Input: part model. Units: mm. Frame: model coordinates. A direction names the side the tool comes from. Round coordinates to 2 decimals unless told otherwise and drop trailing zeros. Loops run counter-clockwise (first coordinate to the right, second up) from the corner with the lowest first, then second, coordinate; pieces in that order, holes last.
(1) Line query: line 1 (X direction, y = -3.5, z = 1.1); line 2 (X direction, y = -6, z = 0.45); line 3 (Y direction, x = 0, z = 1.5). Output: solid intervals per line, ascending.
(2) Cut plane D-D, the plane x = 40. Output: boundary loops of the cut face in (y, z), and give its area (3 significant figures).
(3) Access query for faces 3 (the face through (8, -8, 1)), 4 (the face through (25, -3, 1.5)), 5 (the face through (23, -6, 1)), 6 (the face through (32, 0.1, 0.8)). Directions: +Z, -Z, +X, -X, +Y, -Y. A direction counts if a zero-diameter tool reaches every point of the face in a straight line with its end or side. Return the directions, or none.
(4) Cut plane A-A, the plane y = -6. Output: boundary loops of the cut face in (x, z), and give its area (3 significant figures).
(5) Draft query along X for faces 1 (the face through (9.5, 3, 1.5)), 2 (the face through (-1.97, -4.63, 0.99)). Return one class per face: released by +X, released by -X, zero draft, split by the parting line, or undercut.
(6) Cut plane B-B, the plane z = 1.35. Give the number of separate pieces and of enclosed holes in the cut face, and give its area (3 significant figures).
(7) First-contact query: pin 1 Ø1.6 at (x, y) = (0, 6) entering from -Z; pin 2 Ø1.1 at (x, z) = (21.5, 0.5) entering from -Y; pin 3 Ø0.6 at (y, z) = (-5, 1.5) entering from +X; pin 4 Ø3 at (x, y) = (19.5, -0.5) entering from +Z. Flat tips, straight axial feed; report the tip coordinate or a pass-through.
(8) Cut plane C-C, the plane x = 35. Output: boundary loops of the cut face in (y, z), and give its area (3 significant figures).
from build123d import *

# Parameters (mm, degrees)
CROQUIS1_R              = 0.9
CROQUIS1_R_2            = 1.1
SALIENTE_EXTRUIR1_DEPTH = 2
CROQUIS2_W              = 12
CROQUIS2_H              = 3
CORTAR_EXTRUIR1_DEPTH   = 1
CROQUIS3_W              = 6
CROQUIS3_H              = 10
CORTAR_EXTRUIR2_DEPTH   = 44.194444087


with BuildPart() as part:
    # Croquis1 → Saliente-Extruir1 (new body)
    with BuildSketch(Plane.XY):
        with BuildLine():
            Line((-1.326649916, 8), (20, 8))
            Line((20, 8), (20, 0))
            Line((20, 0), (8, 0))
            Line((8, 0), (8, 4))
            Line((8, 4), (1.326649916, 4))
            ThreePointArc((1.326649916, 4), (-2, 4.673350084), (-1.326649916, 8))
        make_face()
        with Locations((0, 6)):
            Circle(CROQUIS1_R, mode=Mode.SUBTRACT)
        with Locations((12, 3.5)):
            Circle(CROQUIS1_R_2, mode=Mode.SUBTRACT)
    extrude(amount=SALIENTE_EXTRUIR1_DEPTH)

    # Croquis2 → Cortar-Extruir1 (cut)
    with BuildSketch(Plane.XY.offset(2)):
        with Locations((14, 1.5)):
            Rectangle(CROQUIS2_W, CROQUIS2_H)
    extrude(amount=-CORTAR_EXTRUIR1_DEPTH, mode=Mode.SUBTRACT)

    # Simetría1: part across plane


with BuildPart() as part_1:
    add(part.part)
    add(part.part.mirror(Plane(origin=(20, 0, 2), x_dir=(0, 0, 1), z_dir=(0, 1, 0))))

    # Simetría2: part across plane


with BuildPart() as part_2:
    add(part_1.part)
    add(part_1.part.mirror(Plane(origin=(20, 8, 2), x_dir=(0, 0, 1), z_dir=(-1, 0, 0))))

    # Croquis3 → Cortar-Extruir2 (cut, through all)
    with BuildSketch(Plane.XY.offset(2)):
        with Locations((20, -8)):
            Rectangle(CROQUIS3_W, CROQUIS3_H)
    extrude(amount=-CORTAR_EXTRUIR2_DEPTH, mode=Mode.SUBTRACT)


solid = part_2.part
Reported:
1. line 1: x = 8 to 10.9, 13.1 to 17, 23 to 26.9, 29.1 to 32
1. line 2: x = -2.4 to -0.9, 0.9 to 17, 23 to 39.1, 40.9 to 42.4
1. line 3: y = -8 to -6.9, -5.1 to -3.6, 3.6 to 5.1, 6.9 to 8
2. outline: (-8, 0) - (-6.9, 0) - (-6.9, 2) - (-8, 2) - close; (-5.1, 0) - (-3.6, 0) - (-3.6, 2) - (-5.1, 2) - close; (3.6, 0) - (5.1, 0) - (5.1, 2) - (3.6, 2) - close; (6.9, 0) - (8, 0) - (8, 2) - (6.9, 2) - close
2. area: 10.4 mm2
3. face 3: +Z, -Z, +X, -X, -Y
3. face 4: +Z, +X, -X
3. face 5: +Z, -Z, -Y
3. face 6: +Z, -Z
4. outline: (-2.4, 0) - (-0.9, 0) - (-0.9, 2) - (-2.4, 2) - close; (0.9, 0) - (17, 0) - (17, 2) - (0.9, 2) - close; (23, 0) - (39.1, 0) - (39.1, 2) - (23, 2) - close; (40.9, 0) - (42.4, 0) - (42.4, 2) - (40.9, 2) - close
4. area: 70.4 mm2
5. face 1: zero draft
5. face 2: undercut
6. separate pieces: 3
6. enclosed holes: 4
6. area: 352 mm2
7. pin 1: passes through
7. pin 2: stops at y = -3
7. pin 3: stops at x = 42.3
7. pin 4: stops at z = 1
8. outline: (-8, 0) - (-4, 0) - (-4, 2) - (-8, 2) - close; (4, 0) - (8, 0) - (8, 2) - (4, 2) - close
8. area: 16.0 mm2
